Autodesk Inventor part; units mm, degrees
ref_plane "YZ Plane" through (0, 0, 0) normal (1, 0, 0) x (0, 1, 0)
ref_plane "XZ Plane" through (0, 0, 0) normal (0, 1, 0) x (-1, 0, 0)
ref_plane "XY Plane" through (0, 0, 0) normal (0, 0, 1) x (1, 0, 0)
sketch "Sketch1" plane through (0, 0, 0) normal (0, 1, 0) x (-1, 0, 0)
  line L0 (25, 32.5) -> (-25, 32.5)
  line L1 (-25, 32.5) -> (-25, -22.5)
  line L2 (-25, -22.5) -> (25, -22.5)
  line L3 (25, -22.5) -> (25, 32.5)
  circle A0 centre (0, 0) radius 15.2541
  dimension "d0" = 50
  dimension "d1" = 55
  dimension "d2" = 22.5
  dimension "d3" = 25
extrude "Extrusion1" add sketch "Sketch1" along normal blind 150 contours L3 L2 L1 L0 | A0
sketch "Sketch2" plane through (0, 0, 0) normal (0, -1, 0) x (1, 0, 0)
  line L0 (-25, -22.5) -> (-25, 32.5)
  line L1 (-25, 32.5) -> (0, 32.5)
  line L2 (0, 32.5) -> (0, -22.5)
  line L3 (0, -22.5) -> (-25, -22.5)
  line L4 (-25, -22.5) -> (-25, 32.5)
  point P0 (0, 0)
extrude "Extrusion2" cut sketch "Sketch2" against normal blind 50
sketch "Sketch3" plane through (0, 150, 0) normal (0, 1, 0) x (1, 0, 0)
  line L0 (-25, 22.5) -> (-25, -32.5)
  line L1 (25, -32.5) -> (25, 22.5)
  line L2 (-25, -32.5) -> (25, -32.5)
  line L3 (25, -32.5) -> (25, 22.5)
  line L4 (25, 22.5) -> (-25, 22.5)
  line L5 (-25, 22.5) -> (-25, -32.5)
  line L6 (-20, -27.5) -> (20, -27.5)
  line L7 (20, -27.5) -> (20, 17.5)
  line L8 (20, 17.5) -> (-20, 17.5)
  line L9 (-20, 17.5) -> (-20, -27.5)
  point P0 (0, 0)
  dimension "d8" = 5
  dimension "d9" = 5
  dimension "d10" = 5
  dimension "d11" = 5
extrude "Extrusion3" cut sketch "Sketch3" against normal blind 100 contours L9 L8 L7 L6
fillet "Fillet1" radius 3 3 edges at (10, 50, -17.5) (20, 50, 5) (10, 50, 27.5)
sketch "Sketch4" plane through (0, 150, 0) normal (0, 1, 0) x (1, 0, 0)
  line L0 (25, -32.5) -> (25, 22.5)
  line L1 (-25, 22.5) -> (-25, -32.5)
  line L2 (25, -32.5) -> (-25, -32.5)
  line L3 (-25, -32.5) -> (-25, 22.5)
  line L4 (-25, 22.5) -> (25, 22.5)
  line L5 (25, 22.5) -> (25, -32.5)
  point P0 (0, 0)
extrude "Extrusion4" add sketch "Sketch4" against normal blind 7
sketch "Sketch5" plane through (0, 150, 0) normal (0, 1, 0) x (1, 0, 0)
  circle A0 centre (0, 0) radius 6.5
  line L0 (0, -24.5) -> (0, 14.5)
  circle A1 centre (0, -7) radius 15.5
  line L1 (9.6514, -23.7167) -> (0, -7)
  line L2 (0, -7) -> (-9.5909, -23.612)
  line L3 (0, -7) -> (-18.6754, -7)
  line L4 (0, -7) -> (9.4872, 9.4324)
  line L5 (0, -7) -> (16.3511, -7)
  line L6 (0, -7) -> (-10.3523, 10.9308)
  circle A2 centre (15.5, -7) radius 1.5
  circle A3 centre (7.75, -20.4234) radius 1.5
  circle A4 centre (-7.75, -20.4234) radius 1.5
  circle A5 centre (-15.5, -7) radius 1.5
  circle A6 centre (-7.75, 6.4234) radius 1.5
  circle A7 centre (7.75, 6.4234) radius 1.5
  dimension "d17" = 31
  dimension "d18" = 7
  dimension "d19" = 13
  dimension "d20" = 60
  dimension "d21" = 60
  dimension "d22" = 60
  dimension "d23" = 60
  dimension "d24" = 60
  dimension "d25" = 30
  dimension "d26" = 3
  dimension "d27" = 3
  dimension "d28" = 3
  dimension "d29" = 3
  dimension "d30" = 3
  dimension "d31" = 3
extrude "Extrusion5" cut sketch "Sketch5" against normal blind 7 contours A0 L4 | L4 A0 L0 | L0 A0 L6 | A7 A1 L4 | L4 A1 A7 | L6 A0 | L4 A7 A1 | A1 A7 L4 | A3 A1 L1 | L1 A1 A3 | A4 A1 L2 | L2 A1 A4 | A5 A1 L3 | L3 A1 A5 | A2 A1 L5 | L5 A1 A2 | A6 A1 L6 | L6 A1 A6 | A1 L6 A6 | A2 A1 | A4 L2 A1 | A1 L1 A3 | A1 A3 L1 | L2 A4 A1 | L3 A5 A1 | A1 A5 L3 | A1 A6 L6 picked at (1.7263, 1.3919) picked at (-2.6431, 1.1884)
fillet "Fillet2" radius 3 2 edges at (0, 143, -17.5) (0, 143, 27.5)
fillet "Fillet3" radius 3 4 edges at (25, 75, 32.5) (25, 75, -22.5) (-25, 100, -22.5) (-25, 100, 32.5)
sketch "Sketch6" plane through (-25, 50, 29.5) normal (-1, 0, 0) x (0, 0, 1)
  line L0 (-2, 90) -> (-2, 0)
  line L1 (-47, 90) -> (-47, 3)
  line L2 (-2, 90) -> (-47, 90)
  line L3 (-47, 90) -> (-47, 10)
  line L4 (-47, 10) -> (-2, 10)
  line L5 (-2, 10) -> (-2, 90)
  line L6 (-49, 0) -> (0, 0)
  line L7 (-49, 100) -> (0, 100)
  line L8 (-4, 90) -> (-4, 10)
  line L9 (-45, 90) -> (-45, 10)
  line L10 (-52, 100) -> (-52, 0)
  point P0 (-29.5, -50)
  point P1 (3, 0)
  dimension "d36" = 10
  dimension "d38" = 10
  dimension "d39" = 7
  dimension "d40" = 7
extrude "Extrusion6" cut sketch "Sketch6" against normal blind 7 contours L8 L4 L9 L2
fillet "Fillet4" radius 3 4 edges at (-22.5, 140, 25.5) (-22.5, 60, 25.5) (-22.5, 60, -15.5) (-22.5, 140, -15.5)
sketch "Sketch7" plane through (0, 0, -22.5) normal (-1, 0, 0) x (0, 0, 1)
  line L0 (45, 40) -> (10, 40)
  line L1 (10, 40) -> (10, 10)
  line L2 (10, 10) -> (45, 10)
  line L3 (45, 10) -> (45, 40)
  line L4 (55, 50) -> (55, 0)
  line L5 (55, 0) -> (0, 0)
  line L6 (0, 0) -> (0, 50)
  line L7 (3, 50) -> (52, 50)
  circle A0 centre (45, 10) radius 1.95
  circle A1 centre (45, 40) radius 1.95
  circle A2 centre (10, 40) radius 1.95
  circle A3 centre (10, 10) radius 1.95
  point P0 (22.5, 0)
  dimension "d44" = 10
  dimension "d45" = 10
  dimension "d46" = 10
  dimension "d47" = 10
  dimension "d48" = 3.9
  dimension "d49" = 3.9
  dimension "d50" = 3.9
  dimension "d51" = 3.9
extrude "Extrusion7" cut sketch "Sketch7" against normal blind 25 contours A2 L1 L0 | L0 L1 A2 | A1 L3 L0 | L0 L3 A1 | A3 L2 L1 | L1 L2 A3 | A0 L2 L3 | L3 L2 A0
sketch "Sketch8" plane through (25, 0, 29.5) normal (1, 0, 0) x (0, 0, -1)
  circle A0 centre (7, 10) radius 1.95
  circle A1 centre (7, 10) radius 4.5
  circle A2 centre (7, 40) radius 1.95
  circle A3 centre (7, 40) radius 4.5
  circle A4 centre (42, 40) radius 1.95
  circle A5 centre (42, 40) radius 4.5
  circle A6 centre (42, 10) radius 1.95
  circle A7 centre (42, 10) radius 4.5
  point P0 (29.5, 0)
  dimension "d54" = 9
  dimension "d55" = 9
  dimension "d56" = 9
  dimension "d57" = 9
extrude "Extrusion8" cut sketch "Sketch8" against normal blind 10
properties part number "Link2_v2b"
The listing builds one solid part. Answer for the finished solid, in the listing's coordinates (mm). A direction names the side the tool comes from. Round coordinates to 2 decimals unless told otherwise and drop trailing zeros. Write each loop counter-clockwise with the first axis right and the second up, starting at its lowest first coordinate (ties: lowest second). Pieces come first, ordered by that corner, then holes. Notation, with made-up numbers: (10.25, 22.5) -> (34.25, 22.5) arc R34 ccw to (34.25, 60.5) -> close; hole circle Ø1 at (35, -0.75). An arc over 180 degrees is marked (long way). Write item = value, one per line.
1) Straight lines are drawn through the part: line 1 along Z through (x, y) = (8, 10); line 2 along Y through (x, z) = (17, 10.5); line 3 along Y through (x, z) = (22, -12). For each, find the intervals that lie inside material, in ascending order. Write a range as [from, to].
Check values:
line_1 = [-22.5, -14.45], [-10.55, 20.55], [24.45, 32.5]
line_2 = [0, 50], [143, 150]
line_3 = [0, 5.53], [14.47, 35.53], [44.47, 150]
2) Given pin 1 (12.5 mm diameter, centred on x = -14.5, z = 18, fed in from -Y); pin 2 (7 mm diameter, centred on y = 10, z = -12.5, fed in from +X); pin 3 (13.5 mm diameter, centred on y = 82, z = 7.5, fed in from -X); pin 4 (2.5 mm diameter, centred on x = -7.75, z = 20.42, fed in from +Y), each flat-ended and moving along its own axis, determine where each tip first touches the part or whether it passes through.
Check values:
pin_1 = 50
pin_2 = 15
pin_3 = 20
pin_4 = through
3) Section C-C on y = 75.5 is taken. Write down the section's boundary in (x, z), plus the area to 3 significant figures.
Check values:
outline = (-25, -19.5) arc R3 ccw to (-22, -22.5) -> (22, -22.5) arc R3 ccw to (25, -19.5) -> (25, 29.5) arc R3 ccw to (22, 32.5) -> (-22, 32.5) arc R3 ccw to (-25, 29.5) -> (-25, 25.5) -> (-20, 25.5) -> (-20, 27.5) -> (20, 27.5) -> (20, -17.5) -> (-20, -17.5) -> (-20, -15.5) -> (-25, -15.5) -> close
area = 737 mm²
4) Section A-A on y = 10 is taken. Write down the section's boundary in (x, z).
Check values:
outline = (0, -22.5) -> (22, -22.5) arc R3 ccw to (25, -19.5) -> (25, -17) -> (15, -17) -> (15, -14.45) -> (0, -14.45) -> close; (0, -10.55) -> (15, -10.55) -> (15, -8) -> (25, -8) -> (25, 18) -> (15, 18) -> (15, 20.55) -> (0, 20.55) -> close; (0, 24.45) -> (15, 24.45) -> (15, 27) -> (25, 27) -> (25, 29.5) arc R3 ccw to (22, 32.5) -> (0, 32.5) -> close
5) Section D-D on x = -11.5 is taken. Write down the section's boundary in (y, z), plus the area to 3 significant figures.
Check values:
outline = (50, -22.5) -> (150, -22.5) -> (150, 32.5) -> (50, 32.5) -> (50, 27.5) -> (140, 27.5) arc R3 cw to (143, 24.5) -> (143, -14.5) arc R3 cw to (140, -17.5) -> (50, -17.5) -> close
area = 1,320 mm²
6) Which of the six approach directions +Z, -Z, +X, -X, +Y, -Y give full straight-line access (tool end or side, diameter ignored) to faces 1 (the cylindrical face through (9.86, 50.9, -16.64)), 2 (the cylindrical face through (20.07, 11.352, -16.792)), 3 (the flat face through (-23, 140, 5))?
Check values:
face_1 = none
face_2 = +X
face_3 = -X
7) For a pull along Y with two mould halves and no side action, classify faces 4 (the flat face through (-23, 101, 25.5)), 5 (the cylindrical face through (-24.14, 99.3, -21.6)), 6 (the flat face through (-21, 50, 5)) as released by +Y, released by -Y, zero draft, split by the parting line, or undercut.
Check values:
face_4 = undercut
face_5 = zero draft
face_6 = released by -Y
8) Section B-B on x = 11 is taken. Write down the section's boundary in (y, z), plus the area to 3 significant figures.
Check values:
outline = (0, -22.5) -> (150, -22.5) -> (150, 32.5) -> (0, 32.5) -> close; hole circle Ø3.9 at (10, -12.5); hole circle Ø3.9 at (10, 22.5); hole circle Ø3.9 at (40, -12.5); hole circle Ø3.9 at (40, 22.5); hole (50, -14.5) arc R3 ccw to (53, -17.5) -> (140, -17.5) arc R3 ccw to (143, -14.5) -> (143, 24.5) arc R3 ccw to (140, 27.5) -> (53, 27.5) arc R3 ccw to (50, 24.5) -> close
area = 4,020 mm²
